Could you check a few things on this model? Use its own coordinates, in mm. A direction names the side the tool comes from. Round coordinates to 2 decimals unless told otherwise and drop trailing zeros. Loops run counter-clockwise (first coordinate to the right, second up) from the corner with the lowest first, then second, coordinate; pieces in that order, holes last. Notation, with made-up numbers: M 39.5,76 L 71.5,76 A37 cw 71.5,113 Z; hole C 30,23.25 d10. An arc over 180 degrees is marked long. Answer in a Markdown table with one row per item.
```python
from build123d import *

# Parameters (mm, degrees)
SKETCH_1_W          = 65
SKETCH_1_H          = 30
EXTRUDE_1_DEPTH     = 48
SKETCH_2_R          = 1.25
CUT_EXTRUDE_1_DEPTH = 3
SKETCH_3_R          = 7.5
SKETCH_3_R_2        = 1.5
EXTRUDE_2_DEPTH     = 1
SKETCH_4_R          = 1.5
EXTRUDE_3_DEPTH     = 6
CUT_EXTRUDE_START   = -4
SKETCH_5_R          = 1.25
CUT_EXTRUDE_2_DEPTH = 4
EXTRUDE_START       = 1
SKETCH_6_R          = 7.5
SKETCH_6_R_2        = 1.5
EXTRUDE_4_DEPTH     = 1
EXTRUDE_START_2     = 6
SKETCH_7_R          = 1.5
EXTRUDE_5_DEPTH     = 6


with BuildPart() as part:
    # ｽｹｯﾁ1 → ﾎﾞｽ - 押し出し1 (new body)
    with BuildSketch(Plane.XY):
        with Locations((32.5, 15)):
            Rectangle(SKETCH_1_W, SKETCH_1_H)
    extrude(amount=EXTRUDE_1_DEPTH)

    # ｽｹｯﾁ2 → ｶｯﾄ - 押し出し1 (cut)
    with BuildSketch(Plane.XY.offset(48)):
        with Locations((3, 27)):
            Circle(SKETCH_2_R)
        with Locations((15, 27)):
            Circle(SKETCH_2_R)
        with Locations((3, 3)):
            Circle(SKETCH_2_R)
        with Locations((3, 15)):
            Circle(SKETCH_2_R)
        with Locations((15, 3)):
            Circle(SKETCH_2_R)
        with Locations((62, 27)):
            Circle(SKETCH_2_R)
        with Locations((62, 3)):
            Circle(SKETCH_2_R)
    extrude(amount=-CUT_EXTRUDE_1_DEPTH, mode=Mode.SUBTRACT)

    # ｽｹｯﾁ3 → ﾎﾞｽ - 押し出し2 (add)
    with BuildSketch(Plane.XY.offset(48)):
        with Locations(Location((50, 15, 0), (0, 0, 180))):
            Circle(SKETCH_3_R)
        with Locations((50, 15)):
            Circle(SKETCH_3_R_2, mode=Mode.SUBTRACT)
    extrude(amount=EXTRUDE_2_DEPTH)

    # ｽｹｯﾁ4 → ﾎﾞｽ - 押し出し3 (add)
    with BuildSketch(Plane.XY.offset(48)):
        with Locations((50, 15)):
            Circle(SKETCH_4_R)
    extrude(amount=EXTRUDE_3_DEPTH)

    # ｽｹｯﾁ5 → ｶｯﾄ - 押し出し2 (cut)
    with BuildSketch(Plane(origin=(0, 0, 0), x_dir=(-1, 0, 0), z_dir=(0, 0, -1)).offset(CUT_EXTRUDE_START)):
        with Locations(Location((-3, 3, 0), (0, 0, 180))):
            Circle(SKETCH_5_R)
        with Locations(Location((-3, 27, 0), (0, 0, 180))):
            Circle(SKETCH_5_R)
        with Locations((-27, 27)):
            Circle(SKETCH_5_R)
        with Locations((-27, 3)):
            Circle(SKETCH_5_R)
        with Locations(Location((-62, 27, 0), (0, 0, 180))):
            Circle(SKETCH_5_R)
        with Locations(Location((-62, 3, 0), (0, 0, 180))):
            Circle(SKETCH_5_R)
    extrude(amount=CUT_EXTRUDE_2_DEPTH, mode=Mode.SUBTRACT)

    # ｽｹｯﾁ6 → ﾎﾞｽ - 押し出し4 (add)
    with BuildSketch(Plane(origin=(0, 0, 0), x_dir=(-1, 0, 0), z_dir=(0, 0, -1)).offset(EXTRUDE_START)):
        with Locations((-50, 15)):
            Circle(SKETCH_6_R)
        with Locations(Location((-50, 15, 0), (0, 0, 180))):
            Circle(SKETCH_6_R_2, mode=Mode.SUBTRACT)
    extrude(amount=-EXTRUDE_4_DEPTH)

    # ｽｹｯﾁ7 → ﾎﾞｽ - 押し出し5 (add)
    with BuildSketch(Plane(origin=(0, 0, 0), x_dir=(-1, 0, 0), z_dir=(0, 0, -1)).offset(EXTRUDE_START_2)):
        with Locations(Location((-50, 15, 0), (0, 0, 180))):
            Circle(SKETCH_7_R)
    extrude(amount=-EXTRUDE_5_DEPTH)


solid = part.part
```
1) I want a section at A-A, the plane z = 1. Please give me the cut outline in (x, y), plus the area to 3 significant figures.
Computed:
| item | result |
|---|---|
| outline | M 0,0 L 65,0 L 65,30 L 0,30 Z; hole C 3,3 d2.5; hole C 3,27 d2.5; hole C 27,3 d2.5; hole C 27,27 d2.5; hole C 62,3 d2.5; hole C 62,27 d2.5 |
| area | 1,920 mm² |
2) Which directions (+Z, -Z, +X, -X, +Y, -Y) give clear straight access to the entire face, cutting with the end or side of a thin tool? Please do faces 4 (the face through (14.079, 3.845, 46.521)), 5 (the face through (62, 3, 4)).
Computed:
| item | result |
|---|---|
| face 4 | +Z |
| face 5 | -Z |
3) Will these pins go through, and if not, where does the flat tip stop? P1, Ø2, axis at x = 61.5, y = 2.5, coming from the +Z side; P2, Ø2, axis at x = 15, y = 27, coming from the +Z side; P3, Ø4, axis at x = 26.5, y = 16.5, coming from the -Z side.
Computed:
| item | result |
|---|---|
| P1 | stops at z = 48 |
| P2 | stops at z = 45 |
| P3 | stops at z = 0 |
4) I want a section at D-D, the plane x = 50. Please give me the cut outline in (y, z), plus the area to 3 significant figures.
Computed:
| item | result |
|---|---|
| outline | M 0,0 L 7.5,0 L 7.5,-1 L 13.5,-1 L 13.5,-6 L 16.5,-6 L 16.5,-1 L 22.5,-1 L 22.5,0 L 30,0 L 30,48 L 22.5,48 L 22.5,49 L 16.5,49 L 16.5,54 L 13.5,54 L 13.5,49 L 7.5,49 L 7.5,48 L 0,48 Z |
| area | 1,500 mm² |
5) If we mould it in two halves opening along Y, with no side actions, what happens to faces 1 (the face through (32, 0, 24)), 2 (the face through (48.5, 15.07, 51.46)), 3 (the face through (3, 3, 4))? For each: released by +Y, released by -Y, zero draft, split by the parting line, or undercut.
Computed:
| item | result |
|---|---|
| face 1 | released by -Y |
| face 2 | split by the parting line |
| face 3 | undercut |
6) I want a section at C-C, the plane x = 62. Please give me the cut outline in (y, z).
Computed:
| item | result |
|---|---|
| outline | M 0,0 L 1.75,0 L 1.75,4 L 4.25,4 L 4.25,0 L 25.75,0 L 25.75,4 L 28.25,4 L 28.25,0 L 30,0 L 30,48 L 28.25,48 L 28.25,45 L 25.75,45 L 25.75,48 L 4.25,48 L 4.25,45 L 1.75,45 L 1.75,48 L 0,48 Z |
7) I want a section at B-B, the plane y = 15. Please give me the cut outline in (x, z).
Computed:
| item | result |
|---|---|
| outline | M 0,0 L 42.5,0 L 42.5,-1 L 48.5,-1 L 48.5,-6 L 51.5,-6 L 51.5,-1 L 57.5,-1 L 57.5,0 L 65,0 L 65,48 L 57.5,48 L 57.5,49 L 51.5,49 L 51.5,54 L 48.5,54 L 48.5,49 L 42.5,49 L 42.5,48 L 4.25,48 L 4.25,45 L 1.75,45 L 1.75,48 L 0,48 Z |
8) I need wall thicknesses on line 1 (Y direction, x = 62, z = 46.65); line 2 (Z direction, x = 45.5, y = 5); line 3 (Z direction, x = 50, y = 10.5). Which ranges of each line are inside material? Lowest first, please.
Computed:
| item | result |
|---|---|
| line 1 | y = 0 to 1.75, 4.25 to 25.75, 28.25 to 30 |
| line 2 | z = 0 to 48 |
| line 3 | z = -1 to 49 |
